Can you work these out from the drawing? Everything is in mm from the part's minimum corner. A direction names the side the tool comes from. Give positions to 0.01 mm unless a question says otherwise; leave off trailing zeros. Write each loop counter-clockwise with the first axis right and the second up, starting at its lowest first coordinate (ties: lowest second). Pieces come first, ordered by that corner, then holes. Notation, with made-up numbers: (-10, 9.25) - (49, 9.25) arc R29 ccw to (49, 38.25) - close; hole circle Ø5 at (1, 33). An arc over 180 degrees is marked (long way). Use a Markdown table: item, result.
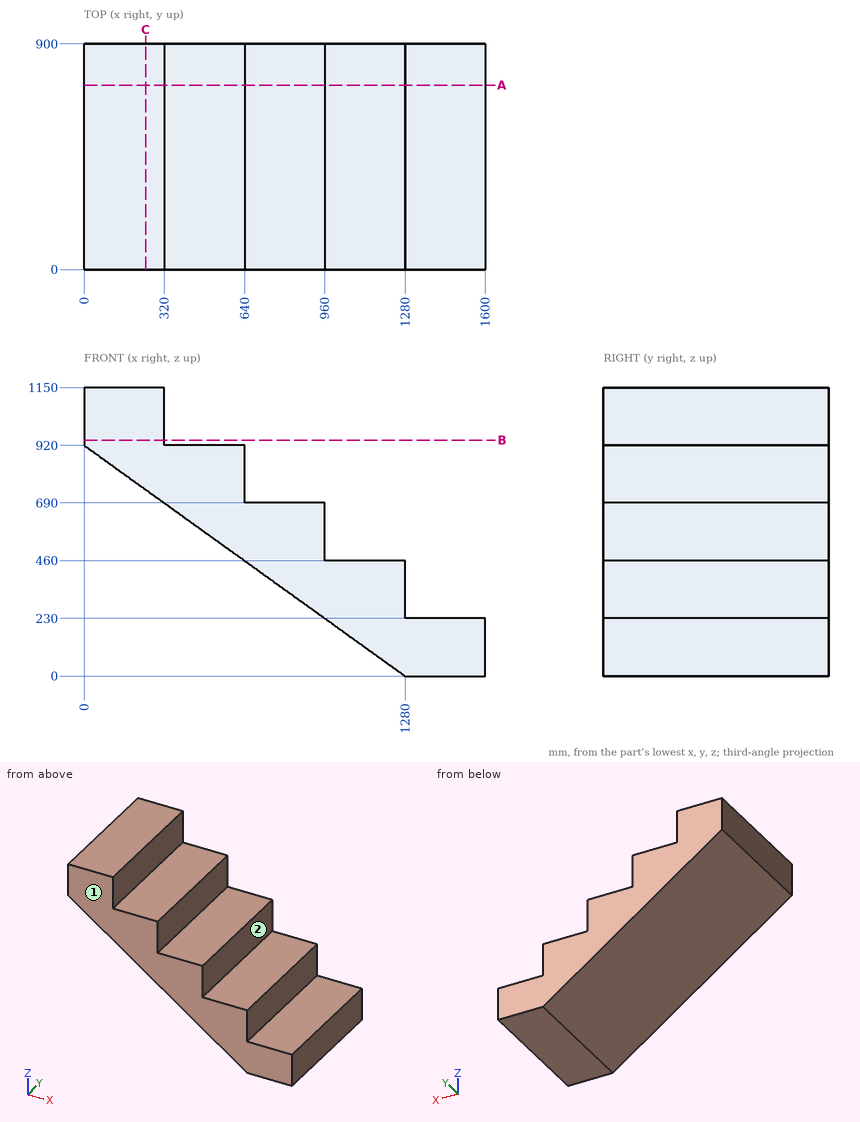
Item 1: I need wall thicknesses on line 1 along Z through (x, y) = (1532, 291.5); line 2 along X through (y, z) = (837, 602); line 3 along X through (y, z) = (75, 565). Which ranges of each line are inside material? Lowest first, please. Write a range as [from, to].
Values:
| item | result |
|---|---|
| line 1 | z = [0, 230] |
| line 2 | x = [442.43, 960] |
| line 3 | x = [493.91, 960] |
Item 2: If we section it at A-A, the plane y = 735.5: Write out the boundary of the cut face in (x, z).
Values:
| item | result |
|---|---|
| outline | (0, 920) - (1280, 0) - (1600, 0) - (1600, 230) - (1280, 230) - (1280, 460) - (960, 460) - (960, 690) - (640, 690) - (640, 920) - (320, 920) - (320, 1150) - (0, 1150) - close |
Item 3: Will these pins go through, and if not, where does the flat tip stop? pin 1 Ø6 at (y, z) = (259.5, 1010.5) entering from +X; pin 2 Ø1.5 at (y, z) = (537, 167.5) entering from -X; pin 3 Ø5 at (y, z) = (327, 246) entering from +X.
Values:
| item | result |
|---|---|
| pin 1 | stops at x = 320 |
| pin 2 | stops at x = 1045.91 |
| pin 3 | stops at x = 1280 |
Item 4: If we section it at B-B, the plane z = 940.5: Write out the boundary of the cut face in (x, y).
Values:
| item | result |
|---|---|
| outline | (0, 0) - (320, 0) - (320, 900) - (0, 900) - close |
Item 5: If we section it at C-C, the plane x = 245.5: Write out the boundary of the cut face in (y, z), plus the area to 3 significant figures.
Values:
| item | result |
|---|---|
| outline | (0, 743.55) - (900, 743.55) - (900, 1150) - (0, 1150) - close |
| area | 366,000 mm2 |
Item 6: For the marked faces 1 and 2, which set-ups out of +Z, -Z, +X, -X, +Y, -Y let a thin tool reach every point of the face, with its end or its side?
Values:
| item | result |
|---|---|
| face 1 | +Z, -Z, +X, -X, -Y |
| face 2 | +Z, +X, +Y, -Y |
